```python
from build123d import *

# Parameters (mm, degrees)
F1_DEPTH = 5
F2_R     = 0.741879
F2_W     = 6.213516
F2_H     = 1.182511
F3_DEPTH = 25
F4_R     = 0.453629
F5_DEPTH = 5.001


with BuildPart() as f1:
    # F0 (on Top) → F1 (new body)
    with BuildSketch(Plane.XY):
        with BuildLine():
            Line((4, 5), (-4, 5))
            ThreePointArc((-4, 5), (-4.707107, 4.707107), (-5, 4))
            Line((-5, 4), (-5, -4))
            ThreePointArc((-5, -4), (-4.707107, -4.707107), (-4, -5))
            Line((-4, -5), (4, -5))
            ThreePointArc((4, -5), (4.707107, -4.707107), (5, -4))
            Line((5, -4), (5, 4))
            ThreePointArc((5, 4), (4.707107, 4.707107), (4, 5))
        make_face()
    extrude(amount=F1_DEPTH)

    # F2 (on face) → F3 (cut)
    with BuildSketch(Plane.XY.offset(5)):
        with Locations((-1.867029, 1.893217)):
            Circle(F2_R)
        with Locations((1.867029, 1.893217)):
            Circle(F2_R)
        with Locations((0, -2.24557)):
            Rectangle(F2_W, F2_H)
    extrude(amount=-F3_DEPTH, mode=Mode.SUBTRACT)

    # F4 (on face) → F5 (cut, through all)
    with BuildSketch(Plane.XY.offset(5)):
        with Locations((-4, 4)):
            Circle(F4_R)
    extrude(amount=-F5_DEPTH, mode=Mode.SUBTRACT)


solid = f1.part
```
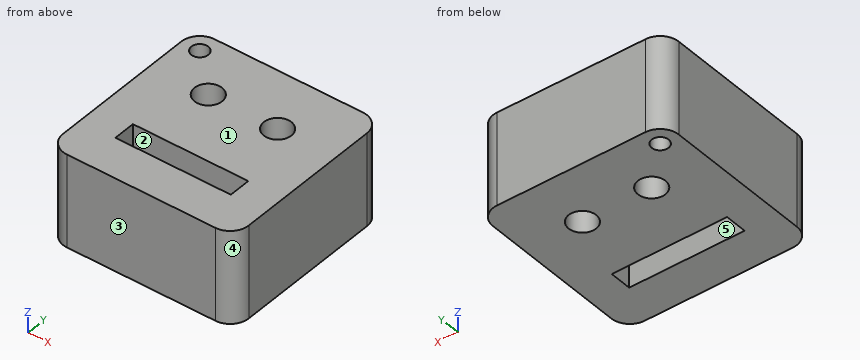
Verification items for the finished model (mm, model axes). Face numbers are marked on the shaded views. A direction names the side the tool comes from. Coordinates: 2 decimals unless noted, no trailing zeros. Write each loop counter-clockwise with the first axis right and the second up, starting at its lowest first coordinate (ties: lowest second). Pieces come first, ordered by that corner, then holes. Notation, with made-up numbers: M 20.25,-7 L 70.25,-7 A21 cw 70.25,28 Z; hole C 3,27.25 d6. An arc over 180 degrees is marked long. Answer as a JSON object with one key per item and string values. Group by question number.
(1) Cross-section at B-B, the plane x = -1.75. Record the cut outline in (y, z).
(2) Cross-section at D-D, the plane y = 4.25. Record the cut outline in (x, z), and give its area (3 significant figures).
(3) Cross-section at A-A, the plane y = 2.25. Record the cut outline in (x, z).
(4) Release check for a two-part mould opening along X. For the marked faces 3, 4 and 5 record: +X half, -X half, draft (parallel to the pull), parting line (faces both ways), or undercut.
(5) Tool access check on the marked faces 1 and 2. Record the directions out of +Z, -Z, +X, -X, +Y, -Y that give a thin tool (end or side, any length) a straight path to the whole face; none if there is none.
(6) Gauge pin test, flat end, axial feed: pin 1 (1 mm diameter, centred on x = 0, y = -4, fed in from -Z). Record the tip position at first contact, or that the pin passes through.
(7) Cross-section at C-C, the plane z = 4.45. Record the cut outline in (x, y), and give its area (3 significant figures).
(8) Material ranges on line 1 (Y direction, x = 0.5, z = 2.5); line 2 (Y direction, x = -4, z = 3.45); line 3 (Y direction, x = 1.75, z = 4.35), recorded low to high.
Reply:
{
 "1": {"outline": "M -5,0 L -2.84,0 L -2.84,5 L -5,5 Z; M -1.65,0 L 1.16,0 L 1.16,5 L -1.65,5 Z; M 2.63,0 L 5,0 L 5,5 L 2.63,5 Z"},
 "2": {"outline": "M -4.97,0 L -4.38,0 L -4.38,5 L -4.97,5 Z; M -3.62,0 L 4.97,0 L 4.97,5 L -3.62,5 Z", "area": "45.9 mm²"},
 "3": {"outline": "M -5,0 L -2.52,0 L -2.52,5 L -5,5 Z; M -1.22,0 L 1.22,0 L 1.22,5 L -1.22,5 Z; M 2.52,0 L 5,0 L 5,5 L 2.52,5 Z"},
 "4": {"face 3": "draft", "face 4": "+X half", "face 5": "undercut"},
 "5": {"face 1": "+Z, +X, -X, +Y, -Y", "face 2": "+Z, -Z"},
 "6": {"pin 1": "z = 0"},
 "7": {"outline": "M -5,-4 A1 ccw -4,-5 L 4,-5 A1 ccw 5,-4 L 5,4 A1 ccw 4,5 L -4,5 A1 ccw -5,4 Z; hole C -4,4 d0.91; hole M -3.11,-2.84 L 3.11,-2.84 L 3.11,-1.65 L -3.11,-1.65 Z; hole C -1.87,1.89 d1.48; hole C 1.87,1.89 d1.48", "area": "87.7 mm²"},
 "8": {"line 1": "-5 to -2.84, -1.65 to 5", "line 2": "-5 to 3.55, 4.45 to 5", "line 3": "-5 to -2.84, -1.65 to 1.16, 2.63 to 5"}
}
